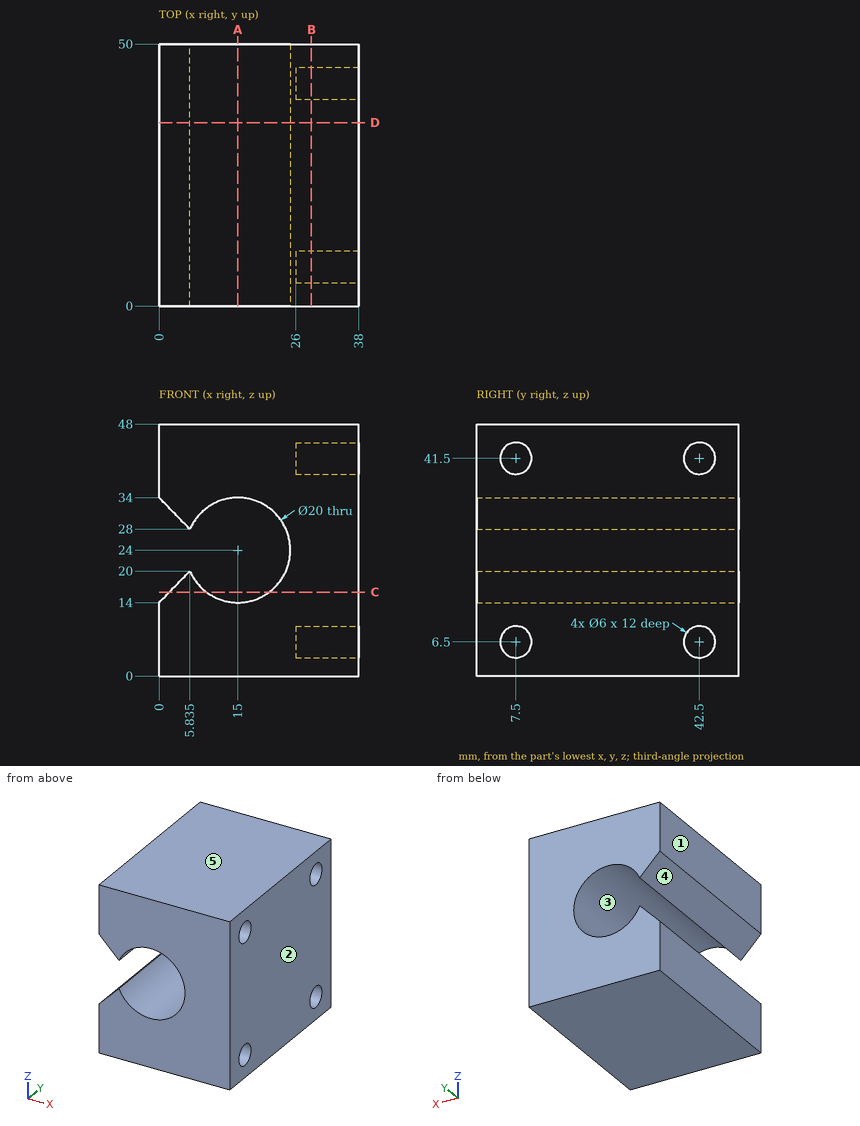
Check sheet for the drawn part. Datum: minimum x, y, z corner. Units: mm. A direction names the side the tool comes from. Round coordinates to 2 decimals unless told otherwise and drop trailing zeros. Order: outer loops, then holes, each group sorted by start corner. A loop starts at its lowest first (then second) coordinate and runs counter-clockwise, first axis right, second up.
(1) Cross-section at A-A, the plane x = 15. Enter the section's corners in (y, z), and give its area (3 significant figures).
(2) Cross-section at B-B, the plane x = 29. Enter the section's corners in (y, z), and give its area (3 significant figures).
(3) Cross-section at C-C, the plane z = 16. Enter the section's corners in (x, y) (3 decimals), and give its area (3 significant figures).
(4) Cross-section at D-D, the plane y = 35. Enter the section's corners in (x, z) (3 decimals).
(5) Scan lines: probe 1 along Z at (x, y) = (15, 15); probe 2 along Z at (x, y) = (29, 42.5); probe 3 along Y at (x, z) = (33, 6). Record each from-to range of solid material in increasing order.
(6) Go/stop test with flat-tipped pins: P1, Ø3, axis at y = 6.5, z = 16, coming from the -X side; P2, Ø18, axis at x = 15, z = 24, coming from the -Y side; P3, Ø3.5, axis at y = 42.5, z = 6.5, coming from the +X side. Record where each tip stops, or that it passes through.
(7) Access from +Z, -Z, +X, -X, +Y, -Y to the whole of each face (thin tool, end or side, straight path). Record for the marked faces 4 and 5.
(8) Draft check along X on the marked faces 1, 2 and 3. Enter one of: pulls with the +X half, pulls with the -X half, needs draft (parallel to the pull), parting line crosses it, or undercut.
Check sheet entries:
1. outline: (0, 0) - (50, 0) - (50, 14) - (0, 14) - close; (0, 34) - (50, 34) - (50, 48) - (0, 48) - close
1. area: 1,400 mm2
2. outline: (0, 0) - (50, 0) - (50, 48) - (0, 48) - close; hole circle Ø6 at (7.5, 6.5); hole circle Ø6 at (7.5, 41.5); hole circle Ø6 at (42.5, 6.5); hole circle Ø6 at (42.5, 41.5)
2. area: 2,290 mm2
3. outline: (1.945, 0) - (9, 0) - (9, 50) - (1.945, 50) - close; (21, 0) - (38, 0) - (38, 50) - (21, 50) - close
3. area: 1,200 mm2
4. outline: (0, 0) - (38, 0) - (38, 48) - (0, 48) - (0, 34) - (5.835, 28) arc R10 cw (long way) to (5.835, 20) - (0, 14) - close
5. probe 1: z = 0 to 14, 34 to 48
5. probe 2: z = 0 to 3.5, 9.5 to 38.5, 44.5 to 48
5. probe 3: y = 0 to 4.54, 10.46 to 39.54, 45.46 to 50
6. P1: stops at x = 0.49
6. P2: passes through
6. P3: stops at x = 26
7. face 4: -X, +Y, -Y
7. face 5: +Z, +X, -X, +Y, -Y
8. face 1: pulls with the -X half
8. face 2: pulls with the +X half
8. face 3: undercut
